Build history of the part. All positions in model axes, mm. Face numbers are marked on the shaded views. Give positions to 0.01 mm unless a question says otherwise; leave off trailing zeros. Write each loop counter-clockwise with the first axis right and the second up, starting at its lowest first coordinate (ties: lowest second). Pieces come first, ordered by that corner, then holes. Notation, with made-up numbers: (7, 51.25) -> (49, 51.25) arc R9 ccw to (49, 61.25) -> close; hole circle Ø2 at (78.5, 28.5). An arc over 180 degrees is marked (long way). Write item = value, one per line. Start each with the question number.
Q1. Drop flat-ended pins along their axis: P1, Ø0.8, axis at y = 0.5, z = -97.5, coming from the -X side; P2, Ø0.8, axis at x = -45, y = 0.5, coming from the +Z side; P3, Ø1.5, axis at y = -0.5, z = 63, coming from the +X side. Give the stop position or say it passes through.
Q2. Mould opens along Z. For the marked faces 1 and 2 say: pulls with the +Z half, pulls with the -Z half, needs draft (parallel to the pull), parting line crosses it, or undercut.
Q3. Wall check: line 1 (Y direction, x = -72.5, z = -120); line 2 (Y direction, x = -60, z = -124); line 3 (Z direction, x = -31.5, y = -1.9). Give the ranges that are in metal, low to high.
Q4. Saw through at A-A, the plane z = -116. List the corners of the cut face in (x, y), then the cut area to 3 significant figures.
Q5. Saw through at B-B, the plane x = -12.5. List the corners of the cut face in (y, z).
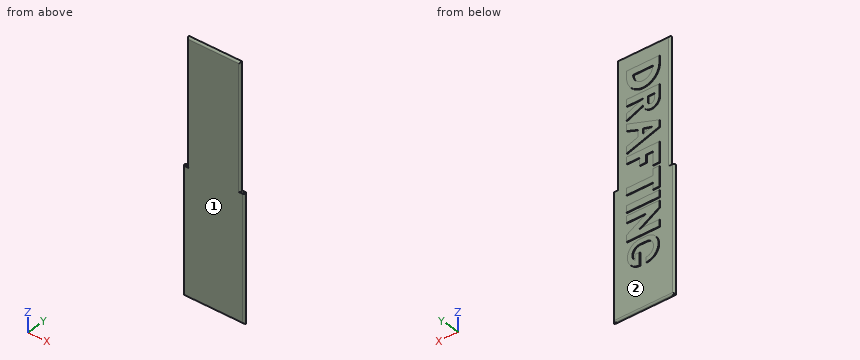
from build123d import *

# Parameters (mm, degrees)
F1_DEPTH    = 4
F2_R        = 1
F3_DEPTH    = 160.54546
F4_T1_DEPTH = 160
F4_T3_DEPTH = 155
F4_T5_DEPTH = 75
F4_T7_DEPTH = 85
F5_R        = 1
F6_DEPTH    = 158.34369
F8_DEPTH    = 1


# Not quite as in the source:
# - a fillet or chamfer that OpenCascade refuses, or shapes differently, is made with other operations: its cross-section is extruded or revolved along the edge and cut away or added


with BuildPart() as f1:
    # F0 (on Front) → F1 (new body)
    with BuildSketch(Plane.XZ):
        Polygon((-75, -3.9577843381), (-75, -153.9577843381), (0, -153.9577843381), (0, -3.9577843381), (-5, -3.9577843381), (-5, 146.0422156619), (-70, 146.0422156619), (-70, -3.9577843381), align=None)
    extrude(amount=F1_DEPTH)

    # F2 (on face) → F3 (cut)
    with BuildSketch(Plane.XY.offset(-3.9577843381)):
        with Locations((-72.5, -2)):
            Circle(F2_R)
    extrude(amount=-F3_DEPTH, mode=Mode.SUBTRACT)

    # F4: fillet of radius 2 on 12 edges, made by hand

    # F4_s2 → F4_t1 (cut)
    with BuildSketch(Plane.XY.offset(-158.9577843381)):
        with BuildLine():
            ThreePointArc((-73, -4), (-74.4142135624, -3.4142135624), (-75, -2))
            Line((-75, -2), (-75, -4))
            Line((-75, -4), (-73, -4))
        make_face()
        with BuildLine():
            ThreePointArc((-73, 0), (-74.4142135624, -0.5857864376), (-75, -2))
            Line((-75, -2), (-75, 0))
            Line((-75, 0), (-73, 0))
        make_face()
        with BuildLine():
            ThreePointArc((-2, 0), (-0.5857864376, -0.5857864376), (0, -2))
            Line((0, -2), (0, 0))
            Line((0, 0), (-2, 0))
        make_face()
        with BuildLine():
            ThreePointArc((-2, -4), (-0.5857864376, -3.4142135624), (0, -2))
            Line((0, -2), (0, -4))
            Line((0, -4), (-2, -4))
        make_face()
    extrude(amount=F4_T1_DEPTH, mode=Mode.SUBTRACT)

    # F4_s4 → F4_t3 (cut)
    with BuildSketch(Plane.XY.offset(-3.9577843381)):
        with BuildLine():
            ThreePointArc((-68, -4), (-69.4142135624, -3.4142135624), (-70, -2))
            Line((-70, -2), (-70, -4))
            Line((-70, -4), (-68, -4))
        make_face()
        with BuildLine():
            ThreePointArc((-68, 0), (-69.4142135624, -0.5857864376), (-70, -2))
            Line((-70, -2), (-70, 0))
            Line((-70, 0), (-68, 0))
        make_face()
        with BuildLine():
            ThreePointArc((-5, -2), (-5.5857864376, -0.5857864376), (-7, 0))
            Line((-7, 0), (-5, 0))
            Line((-5, 0), (-5, -2))
        make_face()
        with BuildLine():
            ThreePointArc((-5, -2), (-5.5857864376, -3.4142135624), (-7, -4))
            Line((-7, -4), (-5, -4))
            Line((-5, -4), (-5, -2))
        make_face()
    extrude(amount=F4_T3_DEPTH, mode=Mode.SUBTRACT)

    # F4_s6 → F4_t5 (cut)
    with BuildSketch(Plane.YZ.offset(-75)):
        with BuildLine():
            ThreePointArc((-2, 146.0422156619), (-3.4142135624, 145.4564292243), (-4, 144.0422156619))
            Line((-4, 144.0422156619), (-4, 146.0422156619))
            Line((-4, 146.0422156619), (-2, 146.0422156619))
        make_face()
        with BuildLine():
            ThreePointArc((-2, 146.0422156619), (-0.5857864376, 145.4564292243), (0, 144.0422156619))
            Line((0, 144.0422156619), (0, 146.0422156619))
            Line((0, 146.0422156619), (-2, 146.0422156619))
        make_face()
    extrude(amount=F4_T5_DEPTH, mode=Mode.SUBTRACT)

    # F4_s8 → F4_t7 (cut)
    with BuildSketch(Plane.YZ.offset(-80)):
        with BuildLine():
            ThreePointArc((-4, -151.9577843381), (-3.4142135624, -153.3719979004), (-2, -153.9577843381))
            Line((-2, -153.9577843381), (-4, -153.9577843381))
            Line((-4, -153.9577843381), (-4, -151.9577843381))
        make_face()
        with BuildLine():
            ThreePointArc((0, -151.9577843381), (-0.5857864376, -153.3719979004), (-2, -153.9577843381))
            Line((-2, -153.9577843381), (0, -153.9577843381))
            Line((0, -153.9577843381), (0, -151.9577843381))
        make_face()
    extrude(amount=F4_T7_DEPTH, mode=Mode.SUBTRACT)

    # F5 (on face) → F6 (cut)
    with BuildSketch(Plane.XY.offset(-3.9577843381)):
        with Locations((-2, -2)):
            Circle(F5_R)
    extrude(amount=-F6_DEPTH, mode=Mode.SUBTRACT)

    # F7 (on face) → F8 (join)
    with BuildSketch(Plane(origin=(0, 0, 0), x_dir=(-1, 0, 0), z_dir=(0, 1, 0))):
        with BuildLine():
            Line((57.5, 127.8843627218), (17.5, 127.8843627218))
            Line((17.5, 127.8843627218), (17.5, 119.8843627218))
            ThreePointArc((17.5, 119.8843627218), (37.5, 99.8843627218), (57.5, 119.8843627218))
            Line((57.5, 119.8843627218), (57.5, 127.8843627218))
        make_face()
        with BuildLine():
            Line((25.5, 119.8843627218), (49.5, 119.8843627218))
            ThreePointArc((49.5, 119.8843627218), (37.5, 107.8843627218), (25.5, 119.8843627218))
        make_face(mode=Mode.SUBTRACT)
        with BuildLine():
            Line((57.5, 95.1502709985), (17.5, 95.1502709985))
            Line((17.5, 95.1502709985), (17.5, 87.1502709985))
            Line((17.5, 87.1502709985), (37.5, 87.1502709985))
            Line((37.5, 87.1502709985), (17.5, 78.7390248019))
            Line((17.5, 78.7390248019), (17.5, 70.7390248019))
            Line((17.5, 70.7390248019), (37.5, 79.1502709985))
            ThreePointArc((37.5, 79.1502709985), (48.4049875621, 71.1003953774), (57.5, 81.1502709985))
            Line((57.5, 81.1502709985), (57.5, 87.1502709985))
            Line((57.5, 87.1502709985), (57.5, 95.1502709985))
        make_face()
        with BuildLine():
            Line((43.5, 87.1502709985), (51.5, 87.1502709985))
            Line((51.5, 87.1502709985), (51.5, 81.1502709985))
            ThreePointArc((51.5, 81.1502709985), (47.5, 77.1502709985), (43.5, 81.1502709985))
            Line((43.5, 81.1502709985), (43.5, 87.1502709985))
        make_face(mode=Mode.SUBTRACT)
        Polygon((57.5, 53.6148357394), (17.5, 66.7390248019), (17.5, 58.7390248019), (31.5839202169, 53.6984175146), (31.5839202169, 45.6984175146), (17.5, 40.7758287685), (17.5, 32.7758287685), (57.5, 45.6148357394), align=None)
        Polygon((37.5, 52.6984175146), (49.1189500386, 49.6984175146), (37.5, 46.6984175146), align=None, mode=Mode.SUBTRACT)
        Polygon((57.5, 28.7758287685), (17.5, 28.7758287685), (17.5, 20.7758287685), (33.5, 20.7758287685), (33.5, 11.7758287685), (41.5, 11.7758287685), (41.5, 20.7758287685), (49.5, 20.7758287685), (49.5, 4.7758287685), (57.5, 4.7758287685), align=None)
        Polygon((57.5, -23.2241712315), (57.5, 0.7758287685), (49.5, 0.7758287685), (49.5, -7.2241712315), (17.5, -7.2241712315), (17.5, -15.2241712315), (49.5, -15.2241712315), (49.5, -23.2241712315), align=None)
        Polygon((57.5, -35.2241712315), (57.5, -27.2241712315), (17.5, -27.2241712315), (17.4124501646, -35.2241712315), align=None)
        Polygon((57.5, -47.2241712315), (57.5, -39.2241712315), (17.5, -39.2241712315), (17.5, -47.2241712315), (41.5822874359, -47.2241712315), (17.5, -61.2241712315), (17.5, -69.2241712315), (57.5, -69.2241712315), (57.5, -61.2241712315), (33.4177125641, -61.2241712315), align=None)
        with BuildLine():
            Line((41.5, -97.2241712315), (41.5, -103.2241712315))
            ThreePointArc((41.5, -103.2241712315), (56.5, -88.2241712315), (41.5, -73.2241712315))
            Line((41.5, -73.2241712315), (33.5, -73.2241712315))
            ThreePointArc((33.5, -73.2241712315), (18.5, -88.2241712315), (33.5, -103.2241712315))
            Line((33.5, -103.2241712315), (33.5, -97.2241712315))
            ThreePointArc((33.5, -97.2241712315), (30.288601192, -96.6317224622), (27.5, -94.932375164))
            ThreePointArc((27.5, -94.932375164), (25.0924487693, -85.0127724236), (33.5, -79.2241712315))
            Line((33.5, -79.2241712315), (41.5, -79.2241712315))
            ThreePointArc((41.5, -79.2241712315), (50.5, -88.2241712315), (41.5, -97.2241712315))
        make_face()
        with BuildLine():
            ThreePointArc((27.5, -94.932375164), (30.288601192, -96.6317224622), (33.5, -97.2241712315))
            Line((33.5, -97.2241712315), (33.5, -88.2241712315))
            Line((33.5, -88.2241712315), (27.5, -88.2241712315))
            Line((27.5, -88.2241712315), (27.5, -94.932375164))
        make_face()
    extrude(amount=F8_DEPTH)


solid = f1.part
Report:
q1.P1 = -53.59
q1.P2 = 127.88
q1.P3 = -5.15
q2.face_1 = needs draft
q2.face_2 = undercut
q3.line_1 = -4 to -3, -1 to 0
q3.line_2 = -4 to 0
q3.line_3 = -153.96 to 146.04
q4.outline = (-73, -4) -> (-2, -4) arc R2 ccw to (-2, 0) -> (-73, 0) arc R2 ccw to start; hole circle Ø2 at (-72.5, -2); hole circle Ø2 at (-2, -2)
q4.area = 290 mm2
q5.outline = (-4, -151.96) arc R2 ccw to (0, -151.96) -> (0, 144.04) arc R2 ccw to (-4, 144.04) -> close
